Check sheet for the modelled part. Datum: model origin and axes. Units: mm. Coordinates: 2 decimals unless noted, no trailing zeros. Loops run counter-clockwise (first coordinate to the right, second up) from the corner with the lowest first, then second, coordinate; pieces in that order, holes last. Notation, with made-up numbers: (-29.75, 8) - (20.25, 8) arc R21 ccw to (20.25, 23) - close; hole circle Ø3 at (43, 72.5). An arc over 180 degrees is marked (long way). Use a Markdown table: item, result. Add a question column.
1) Sectioned sample at C-C, the plane y = 2. Enter the section's corners in (x, z).
2) Thickness scan on line 1 (X direction, y = 2.65, z = 12); line 2 (Z direction, x = -9, y = 3.15); line 3 (X direction, y = 5, z = 14). Record the ranges inside material, lowest first.
3) Sectioned sample at A-A, the plane x = 9. Enter the section's corners in (y, z).
4) Sectioned sample at B-B, the plane z = 12. Enter the section's corners in (x, y), then the cut area to 3 significant figures.
5) Go/stop test with a flat-tipped pin: P1, Ø1.5, axis at x = 0, z = 3, coming from the -Y side. Record where the tip stops, or that it passes through.
from build123d import *

# Parameters (mm, degrees)
SKETCH1_W           = 31
SKETCH1_H           = 35
BOSS_EXTRUDE1_DEPTH = 6
SKETCH2_R           = 2.2
CUT_EXTRUDE1_DEPTH  = 7
FILLET1_R           = 1
CHAMFER1_SIZE       = 0.8


with BuildPart() as part:
    # Sketch1 → Boss-Extrude1 (new body)
    with BuildSketch(Plane(origin=(0, 0, 0), x_dir=(1, 0, 0), z_dir=(0, 1, 0))):
        Rectangle(SKETCH1_W, SKETCH1_H)
    extrude(amount=BOSS_EXTRUDE1_DEPTH)

    # Sketch2 → Cut-Extrude1 (cut, through all)
    with BuildSketch(Plane(origin=(0, 6, 0), x_dir=(1, 0, 0), z_dir=(0, 1, 0))):
        with Locations((9, 12)):
            Circle(SKETCH2_R)
        with Locations((9, -12)):
            Circle(SKETCH2_R)
        with Locations((-9, 12)):
            Circle(SKETCH2_R)
        with Locations((-9, -12)):
            Circle(SKETCH2_R)
    extrude(amount=-CUT_EXTRUDE1_DEPTH, mode=Mode.SUBTRACT)

    # Fillet1
    fillet1_edges = [part.edges().sort_by_distance(p)[0] for p in [
        (15.5, 3, 17.5),
        (-15.5, 3, 17.5),
        (-15.5, 3, -17.5),
        (15.5, 3, -17.5),
    ]]
    fillet(fillet1_edges, radius=FILLET1_R)

    # Chamfer1
    chamfer1_edges = [part.edges().sort_by_distance(p)[0] for p in [
        (6.8, 0, 12),
        (6.8, 6, 12),
        (-11.2, 0, -12),
        (-11.2, 6, -12),
        (-11.2, 0, 12),
        (-11.2, 6, 12),
        (6.8, 0, -12),
        (6.8, 6, -12),
        (0, 0, 17.5),
        (0, 6, 17.5),
        (15.5, 0, 0),
        (-15.5, 0, 0),
        (0, 0, -17.5),
        (15.207106781, 0, 17.207106781),
        (15.207106781, 0, -17.207106781),
        (-15.207106781, 0, -17.207106781),
        (-15.207106781, 0, 17.207106781),
        (-15.5, 6, 0),
        (15.5, 6, 0),
        (0, 6, -17.5),
        (15.207106781, 6, 17.207106781),
        (15.207106781, 6, -17.207106781),
        (-15.207106781, 6, -17.207106781),
        (-15.207106781, 6, 17.207106781),
    ]]
    chamfer(chamfer1_edges, length=CHAMFER1_SIZE)


solid = part.part
Solved:
| question | item | result |
|---|---|---|
| 1 | outline | (-15.5, -16.5) arc R1 ccw to (-14.5, -17.5) - (14.5, -17.5) arc R1 ccw to (15.5, -16.5) - (15.5, 16.5) arc R1 ccw to (14.5, 17.5) - (-14.5, 17.5) arc R1 ccw to (-15.5, 16.5) - close; hole circle Ø4.4 at (-9, -12); hole circle Ø4.4 at (-9, 12); hole circle Ø4.4 at (9, -12); hole circle Ø4.4 at (9, 12) |
| 2 | line 1 | x = -15.5 to -11.2, -6.8 to 6.8, 11.2 to 15.5 |
| 2 | line 2 | z = -17.5 to -14.2, -9.8 to 9.8, 14.2 to 17.5 |
| 2 | line 3 | x = -15.5 to -9.92, -8.08 to 8.08, 9.92 to 15.5 |
| 3 | outline | (0, -16.7) - (0.8, -17.5) - (5.2, -17.5) - (6, -16.7) - (6, -15) - (5.2, -14.2) - (0.8, -14.2) - (0, -15) - close; (0, -9) - (0.8, -9.8) - (5.2, -9.8) - (6, -9) - (6, 9) - (5.2, 9.8) - (0.8, 9.8) - (0, 9) - close; (0, 15) - (0.8, 14.2) - (5.2, 14.2) - (6, 15) - (6, 16.7) - (5.2, 17.5) - (0.8, 17.5) - (0, 16.7) - close |
| 4 | outline | (-15.5, 0.8) - (-14.7, 0) - (-12, 0) - (-11.2, 0.8) - (-11.2, 5.2) - (-12, 6) - (-14.7, 6) - (-15.5, 5.2) - close; (-6.8, 0.8) - (-6, 0) - (6, 0) - (6.8, 0.8) - (6.8, 5.2) - (6, 6) - (-6, 6) - (-6.8, 5.2) - close; (11.2, 0.8) - (12, 0) - (14.7, 0) - (15.5, 0.8) - (15.5, 5.2) - (14.7, 6) - (12, 6) - (11.2, 5.2) - close |
| 4 | area | 129 mm2 |
| 5 | P1 | stops at y = 0 |
